```python
from build123d import *

# Parameters (mm, degrees)
SKETCH1_W          = 330.2
SKETCH1_H          = 47.625
SKETCH1_R          = 12.7
SKETCH1_R_2        = 1.27
EXTRUDE1_DEPTH     = 6.35
CUT_EXTRUDE1_DEPTH = 167.929229484


with BuildPart() as part:
    # Sketch1 → Extrude1 (new body)
    with BuildSketch(Plane.XY):
        Rectangle(SKETCH1_W, SKETCH1_H)
        with Locations((-136.525, 9.8425)):
            Circle(SKETCH1_R, mode=Mode.SUBTRACT)
        with Locations((-95.25, 9.8425)):
            Circle(SKETCH1_R, mode=Mode.SUBTRACT)
        with Locations(Location((95.25, 9.8425, 0), (0, 0, 180))):
            Circle(SKETCH1_R, mode=Mode.SUBTRACT)
        with Locations(Location((136.525, 9.8425, 0), (0, 0, 180))):
            Circle(SKETCH1_R, mode=Mode.SUBTRACT)
        with Locations((59.182, 17.7673)):
            Circle(SKETCH1_R_2, mode=Mode.SUBTRACT)
        with Locations((59.182, 3.4671)):
            Circle(SKETCH1_R_2, mode=Mode.SUBTRACT)
        with BuildLine():
            Line((-54.356, 17.78), (-0.254, 17.78))
            ThreePointArc((-0.254, 17.78), (0.823630735, 17.333630735), (1.27, 16.256))
            Line((1.27, 16.256), (1.27, 3.429))
            ThreePointArc((1.27, 3.429), (0.823630735, 2.351369265), (-0.254, 1.905))
            Line((-0.254, 1.905), (-54.356, 1.905))
            ThreePointArc((-54.356, 1.905), (-55.433630735, 2.351369265), (-55.88, 3.429))
            Line((-55.88, 3.429), (-55.88, 16.256))
            ThreePointArc((-55.88, 16.256), (-55.433630735, 17.333630735), (-54.356, 17.78))
        make_face(mode=Mode.SUBTRACT)
        with BuildLine():
            Line((10.2235, 17.78), (48.4505, 17.78))
            ThreePointArc((48.4505, 17.78), (49.528130735, 17.333630735), (49.9745, 16.256))
            Line((49.9745, 16.256), (49.9745, 3.429))
            ThreePointArc((49.9745, 3.429), (49.528130735, 2.351369265), (48.4505, 1.905))
            Line((48.4505, 1.905), (10.2235, 1.905))
            ThreePointArc((10.2235, 1.905), (9.145869265, 2.351369265), (8.6995, 3.429))
            Line((8.6995, 3.429), (8.6995, 16.256))
            ThreePointArc((8.6995, 16.256), (9.145869265, 17.333630735), (10.2235, 17.78))
        make_face(mode=Mode.SUBTRACT)
    extrude(amount=EXTRUDE1_DEPTH)

    # Sketch2 → Cut-Extrude1 (cut, through all)
    with BuildSketch(Plane.XY):
        Polygon((-167.77348356, 39.759180653), (-167.77348356, -38.14883308), (-131.444750208, -38.14883308), align=None)
    extrude(amount=CUT_EXTRUDE1_DEPTH, mode=Mode.SUBTRACT)


solid = part.part
```
Geometry: final body of the model. Coordinates: model frame, mm. A direction names the side the tool comes from. Coordinates: 2 decimals unless noted, no trailing zeros. Order: outer loops, then holes, each group sorted by start corner. A loop starts at its lowest first (then second) coordinate and runs counter-clockwise, first axis right, second up. Notation, with made-up numbers: (37.25, 40.25) -> (88.25, 40.25) arc R5 ccw to (88.25, 47.25) -> close; hole circle Ø1 at (66.5, -16.5). An arc over 180 degrees is marked (long way). Write each question's results on one line, items separated by ' | '. Start each with the question number.
1) First-contact query: pin 1 (23 mm diameter, centred on x = -136.52, y = 9.84, fed in from +Z); pin 2 (1.9 mm diameter, centred on y = 7.5, z = 2, fed in from -X). Flat tips, straight axial feed; report the tip coordinate or a pass-through.
2) Material intervals for line 1 along Y through (x, z) = (-95.25, 5.25); line 2 along Y through (x, z) = (-6, 2) (1 decimal); line 3 along X through (y, z) = (-18.5, 3.75), sorted ascending.
3) Cut plane D-D, the plane y = -18.5. Output: boundary loops of the cut face in (x, z).
4) Mould query, pull axis Y, two halves, no side actions, for faces 3 (the flat face through (29, 17.78, 3)), 4 (the flat face through (-27, 1.905, 3)), 5 (the flat face through (11, -23.812, 3)), 6 (the flat face through (0, 0, 6.35)). Classes: released by +Y, released by -Y, zero draft, split by the parting line, or undercut.
5) Cut plane A-A, the plane x = 95.25. Output: boundary loops of the cut face in (y, z), and give its area (3 significant figures).
6) Set-up query: faces 1 (the flat face through (-149.08, -0.33, 3.13)), 2 (the flat face through (8.7, 10, 3)). Return all of +Z, -Z, +X, -X, +Y, -Y with unobstructed straight access to the full face (end or side cutting, diameter ignored); none if empty.
7) Cut plane B-B, the plane z = 2.5. State how many separate pieces and enclosed holes the cut face has, and give its area (3 significant figures).
Checks:
1) pin 1: through | pin 2: x = -153.17
2) line 1: -23.81 to -2.86, 22.54 to 23.81 | line 2: -23.8 to 1.9, 17.8 to 23.8 | line 3: -140.61 to 165.1
3) outline: (-140.61, 0) -> (165.1, 0) -> (165.1, 6.35) -> (-140.61, 6.35) -> close
4) face 3: undercut | face 4: undercut | face 5: released by -Y | face 6: zero draft
5) outline: (-23.81, 0) -> (-2.86, 0) -> (-2.86, 6.35) -> (-23.81, 6.35) -> close; (22.54, 0) -> (23.81, 0) -> (23.81, 6.35) -> (22.54, 6.35) -> close | area: 141 mm^2
6) face 1: +Z, -Z, -X, -Y | face 2: +Z, -Z
7) separate pieces: 1 | enclosed holes: 8 | area: 11,400 mm^2
